Can you work these out from the model? Positions are in its coordinate system, mm. Face numbers are marked on the shaded views. A direction names the side the tool comes from. Coordinates: 2 decimals unless noted, no trailing zeros. Write each loop counter-clockwise with the first axis right and the second up, starting at its lowest first coordinate (ties: lowest second). Pieces come first, ordered by that corner, then holes. Notation, with made-up numbers: (42.25, 43) - (90.25, 43) arc R30 cw to (90.25, 74) - close; hole circle Ø9 at (-7, -6.75). An arc over 180 degrees is marked (long way). Use one line per item in the form item = value. Start each with the question number.
(1) If we section it at C-C on z = 4: Please give me the cut outline in (x, y), then the cut area to 3 significant figures.
(2) On a 3-axis mill with a long thin cutter (end or side, diameter ignored), from which of +Z, -Z, +X, -X, +Y, -Y can I reach the whole of each face in a straight line? I mean the marked faces 1 and 2. Say none if no direction works.
(3) For pin 1 Ø1.7 at (x, z) = (-2.5, 3) entering from -Y; pin 2 Ø8 at (x, y) = (-8, -9.5) entering from -Z; pin 3 Ø1 at (x, y) = (8, 5) entering from +Z; pin 4 Ø2.5 at (y, z) = (-13, 3.5) entering from +X, each with a flat end and sliding along its axis, tell me the tip position at first contact or that it passes through.
(4) If we section it at D-D on y = 5: Please give me the cut outline in (x, z).
(5) If we section it at B-B on y = -14: Please give me the cut outline in (x, z).
(6) If I drill on probe 1 along Z at (x, y) = (8.25, -7.5); probe 2 along X at (y, z) = (-11, 3.7); probe 3 along Y at (x, z) = (4, 2.3), over which ranges is the centre line in solid material (lowest first)? Write a range as from..to.
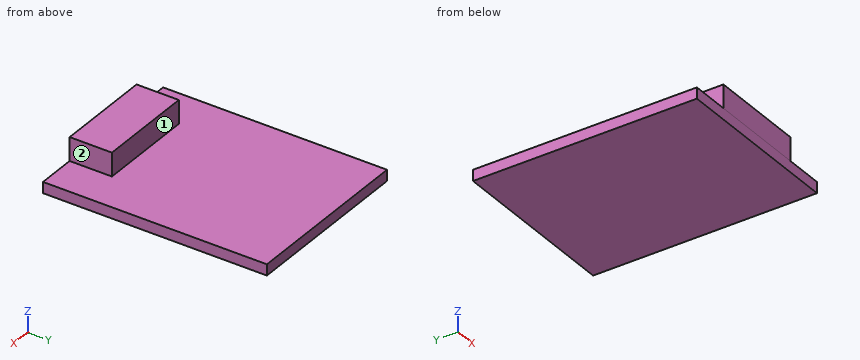
```python
from build123d import *

# Parameters (mm, degrees)
SKETCH_1_W      = 25.5
SKETCH_1_H      = 32.5
EXTRUDE_1_DEPTH = 1.6
SKETCH_2_W      = 14.2
SKETCH_2_H      = 6.13
EXTRUDE_3_DEPTH = 5


with BuildPart() as part:
    # 草图1 → 凸台-拉伸1 (new body)
    with BuildSketch(Plane.XY):
        Rectangle(SKETCH_1_W, SKETCH_1_H)
    extrude(amount=EXTRUDE_1_DEPTH)

    # 草图2 → 凸台-拉伸3 (add)
    with BuildSketch(Plane.XY):
        with Locations((0, -13.175)):
            Rectangle(SKETCH_2_W, SKETCH_2_H)
    extrude(amount=EXTRUDE_3_DEPTH)


solid = part.part
```
Reported:
q1.outline = (-7.1, -16.24) - (7.1, -16.24) - (7.1, -10.11) - (-7.1, -10.11) - close
q1.area = 87.0 mm2
q2.face_1 = +Z, +X, -X, +Y
q2.face_2 = +Z, +X, +Y, -Y
q3.pin_1 = -16.24
q3.pin_2 = 0
q3.pin_3 = 1.6
q3.pin_4 = 7.1
q4.outline = (-12.75, 0) - (12.75, 0) - (12.75, 1.6) - (-12.75, 1.6) - close
q5.outline = (-12.75, 0) - (12.75, 0) - (12.75, 1.6) - (7.1, 1.6) - (7.1, 5) - (-7.1, 5) - (-7.1, 1.6) - (-12.75, 1.6) - close
q6.probe_1 = 0..1.6
q6.probe_2 = -7.1..7.1
q6.probe_3 = -16.24..-10.11
